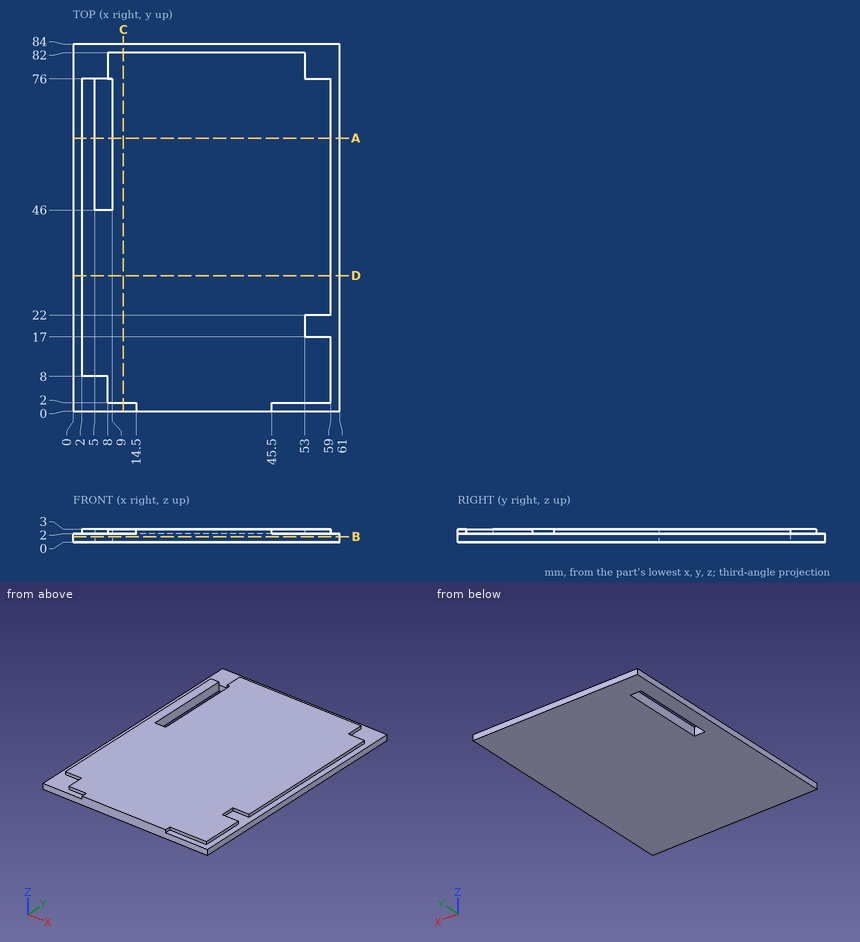
Check sheet for the drawn part. Datum: minimum x, y, z corner. Units: mm. Give positions to 0.01 mm unless a question says otherwise; leave off trailing zeros. Loops run counter-clockwise (first coordinate to the right, second up) from the corner with the lowest first, then second, coordinate; pieces in that order, holes last. Notation, with made-up numbers: (60.5, 18) - (119.5, 18) arc R21 ccw to (119.5, 48) - close; hole circle Ø11 at (55.25, 28). An arc over 180 degrees is marked (long way). Write each question's results on one line, items separated by ' | '.
1) Material ranges on L1, parallel to X at y = 57, z = 2.4; L2, parallel to X at y = 75, z = 1.9; L3, parallel to Y at x = 40, z = 2.1, recorded low to high. Write a range as from..to.
Solution:
L1: 2..5, 9..59 | L2: 0..5, 9..61 | L3: 0..82
2) Sectioned sample at A-A on y = 62.5. Record the boundary of the cut face in (x, z).
Solution:
outline: (0, 0) - (5, 0) - (5, 3) - (2, 3) - (2, 2) - (0, 2) - close; (9, 0) - (61, 0) - (61, 2) - (59, 2) - (59, 3) - (9, 3) - close
3) Sectioned sample at C-C on x = 11.5. Record the boundary of the cut face in (y, z), plus the area to 3 significant figures.
Solution:
outline: (0, 0) - (84, 0) - (84, 2) - (82, 2) - (82, 3) - (2, 3) - (2, 2) - (0, 2) - close | area: 248 mm2
4) Depth check by flat-ended pin: P1, Ø0.5, axis at x = 31.5, z = 2.5, coming from the +Y side; P2, Ø0.8, axis at x = 11.5, z = 2.5, coming from the -Y side; P3, Ø0.5, axis at y = 10, z = 2.5, coming from the +X side. Enter the tip coordinate at first touch or a pass-through.
Solution:
P1: y = 82 | P2: y = 2 | P3: x = 59
5) Sectioned sample at B-B on z = 1.3. Record the boundary of the cut face in (x, y), plus the area to 3 significant figures.
Solution:
outline: (0, 0) - (61, 0) - (61, 84) - (0, 84) - close; hole (5, 46) - (9, 46) - (9, 76) - (5, 76) - close | area: 5,000 mm2
6) Sectioned sample at D-D on y = 31. Record the boundary of the cut face in (x, z), plus the area to 3 significant figures.
Solution:
outline: (0, 0) - (61, 0) - (61, 2) - (59, 2) - (59, 3) - (2, 3) - (2, 2) - (0, 2) - close | area: 179 mm2
